```python
from build123d import *

# Parameters (mm, degrees)
SKETCH1_W           = 130
SKETCH1_H           = 50
BOSS_EXTRUDE1_DEPTH = 40
SKETCH2_W           = 80.3
SKETCH2_H           = 40
CUT_EXTRUDE1_DEPTH  = 51
SKETCH3_R           = 4.1
CUT_EXTRUDE2_DEPTH  = 41
CHAMFER1_SIZE       = 1
SKETCH5_R           = 4.1
CUT_EXTRUDE3_DEPTH  = 41


with BuildPart() as part:
    # Sketch1 → Boss-Extrude1 (new body)
    with BuildSketch(Plane(origin=(0, 0, 0), x_dir=(1, 0, 0), z_dir=(0, 1, 0))):
        Rectangle(SKETCH1_W, SKETCH1_H)
    extrude(amount=BOSS_EXTRUDE1_DEPTH)

    # Sketch2 → Cut-Extrude1 (cut, through all)
    with BuildSketch(Plane.XY.offset(25)):
        with Locations((0, 40)):
            Rectangle(SKETCH2_W, SKETCH2_H)
    extrude(amount=-CUT_EXTRUDE1_DEPTH, mode=Mode.SUBTRACT)

    # Sketch3 → Cut-Extrude2 (cut, through all)
    with BuildSketch(Plane.XZ):
        with Locations((-35, 15)):
            Circle(SKETCH3_R)
        with Locations((-35, -15)):
            Circle(SKETCH3_R)
        with Locations((35, -14.217273236)):
            Circle(SKETCH3_R)
        with Locations((35, 15)):
            Circle(SKETCH3_R)
    extrude(amount=-CUT_EXTRUDE2_DEPTH, mode=Mode.SUBTRACT)

    # Chamfer1
    chamfer1_edges = [part.edges().sort_by_distance(p)[0] for p in [
        (40.15, 40, 0),
        (-40.15, 40, 0),
    ]]
    chamfer(chamfer1_edges, length=CHAMFER1_SIZE)

    # Sketch5 → Cut-Extrude3 (cut, through all)
    with BuildSketch(Plane.XZ):
        with Locations((-55, 15)):
            Circle(SKETCH5_R)
        with Locations((-55, -15)):
            Circle(SKETCH5_R)
        with Locations((55, 15)):
            Circle(SKETCH5_R)
        with Locations((55, -15)):
            Circle(SKETCH5_R)
    extrude(amount=-CUT_EXTRUDE3_DEPTH, mode=Mode.SUBTRACT)


solid = part.part
```
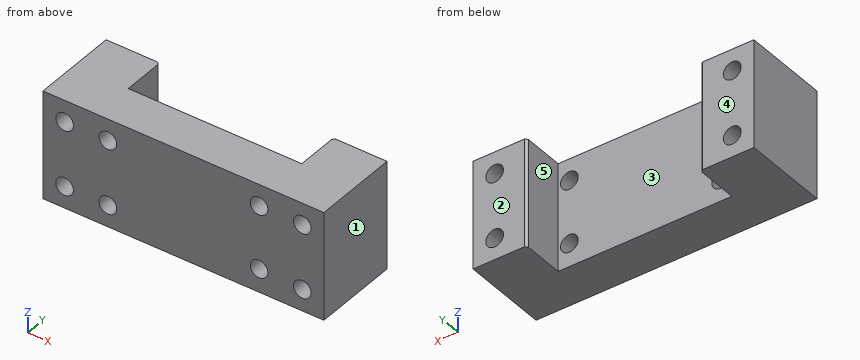
CAD build for the part. Positions are in the model's coordinates, mm. Face numbers are marked on the shaded views. A direction names the side the tool comes from. Round coordinates to 2 decimals unless told otherwise and drop trailing zeros. Loops run counter-clockwise (first coordinate to the right, second up) from the corner with the lowest first, then second, coordinate; pieces in that order, holes last. Notation, with made-up numbers: (25.25, 87.25) - (34.25, 87.25) arc R11 cw to (34.25, 92.25) - close; hole circle Ø11 at (88.25, 85). An arc over 180 degrees is marked (long way). Return JSON: item names as keys, results as strings. Group by question number.
Q1. Tool access for the marked faces 4 and 5: list every direction of +Z, -Z, +X, -X, +Y, -Y with a clear straight run to the whole face (end or side of a thin tool).
Q2. Two-plate mould, pull along X, no slides. Class the marked faces 1, 2 and 3: +X half, -X half, draft (parallel to the pull), parting line (faces both ways), or undercut.
Q3. Band-saw the part on B-B on z = 15. Give the cut face in (x, y), plus the area to 3 significant figures.
Q4. Flat gauge pins, fed straight in: pin 1 Ø12 at (x, z) = (-5, 4) entering from -Y; pin 2 Ø9.5 at (x, z) = (35, 15) entering from +Y. Where does each tip first touch, or does it go through?
Q5. Band-saw the part on D-D on x = -55. Give the cut face in (y, z).
Q6. Drill centre lines: line 1 along Z through (x, y) = (-35, 12); line 2 along Z through (x, y) = (35, 14.5); line 3 along X through (y, z) = (33.5, 17.5). Where is each one in solid material? Low to high. Write a range as [from, to].
Q7. Band-saw the part on C-C on x = -35. Give the cut face in (y, z).
Q8. Band-saw the part on A-A on y = 30. Give the cut face in (x, z), plus the area to 3 significant figures.
Solutions:
{
 "1": {"face 4": "+Z, -Z, +X, -X, +Y", "face 5": "+Z, -Z, +Y"},
 "2": {"face 1": "+X half", "face 2": "draft", "face 3": "undercut"},
 "3": {"outline": "(-65, 0) - (-59.1, 0) - (-59.1, 40) - (-65, 40) - close; (-50.9, 0) - (-39.1, 0) - (-39.1, 20) - (-40.15, 20) - (-40.15, 39) - (-41.15, 40) - (-50.9, 40) - close; (-30.9, 0) - (30.9, 0) - (30.9, 20) - (-30.9, 20) - close; (39.1, 0) - (50.9, 0) - (50.9, 40) - (41.15, 40) - (40.15, 39) - (40.15, 20) - (39.1, 20) - close; (59.1, 0) - (65, 0) - (65, 40) - (59.1, 40) - close", "area": "2,610 mm^2"},
 "4": {"pin 1": "stops at y = 0", "pin 2": "stops at y = 20"},
 "5": {"outline": "(0, -25) - (40, -25) - (40, -19.1) - (0, -19.1) - close; (0, -10.9) - (40, -10.9) - (40, 10.9) - (0, 10.9) - close; (0, 19.1) - (40, 19.1) - (40, 25) - (0, 25) - close"},
 "6": {"line 1": "z = [-25, -19.1], [-10.9, 10.9], [19.1, 25]", "line 2": "z = [-25, -18.32], [-10.12, 10.9], [19.1, 25]", "line 3": "x = [-65, -58.25], [-51.75, -40.15], [40.15, 51.75], [58.25, 65]"},
 "7": {"outline": "(0, -25) - (20, -25) - (20, -19.1) - (0, -19.1) - close; (0, -10.9) - (20, -10.9) - (20, 10.9) - (0, 10.9) - close; (0, 19.1) - (20, 19.1) - (20, 25) - (0, 25) - close"},
 "8": {"outline": "(-65, -25) - (-40.15, -25) - (-40.15, 25) - (-65, 25) - close; (40.15, -25) - (65, -25) - (65, 25) - (40.15, 25) - close; hole circle Ø8.2 at (-55, -15); hole circle Ø8.2 at (-55, 15); hole circle Ø8.2 at (55, -15); hole circle Ø8.2 at (55, 15)", "area": "2,270 mm^2"}
}
